Autodesk Inventor part; units mm, degrees
ref_plane "YZ Plane" through (0, 0, 0) normal (1, 0, 0) x (0, 1, 0)
ref_plane "XZ Plane" through (0, 0, 0) normal (0, 1, 0) x (-1, 0, 0)
ref_plane "XY Plane" through (0, 0, 0) normal (0, 0, 1) x (1, 0, 0)
sketch "Sketch4" plane through (0, 0, 0) normal (0, 0, 1) x (1, 0, 0)
  line L0 (-45, -45) -> (45, -45)
  line L1 (45, -45) -> (45, 45)
  line L2 (45, 45) -> (-45, 45)
  line L3 (-45, 45) -> (-45, -45)
  line L4 (-45, -45) -> (45, 45) construction
  line L5 (45, -45) -> (-45, 45) construction
  point P0 (0, 0)
  dimension "d10" = 90
  dimension "d11" = 90
extrude "Extrusion4" add sketch "Sketch4" along normal blind 12.47
sketch "Sketch5" plane through (0, 0, 12.47) normal (0, 0, 1) x (1, 0, 0)
  line L0 (-45, -45) -> (45, -45)
  line L1 (45, -45) -> (45, 45)
  line L2 (45, 45) -> (-45, 45)
  line L3 (-45, 45) -> (-45, -45)
  line L4 (-45, -45) -> (45, 45) construction
  line L5 (45, -45) -> (-45, 45) construction
  line L6 (45, 45) -> (-45, 45)
  line L7 (45, -45) -> (45, 45)
  circle A0 centre (0, 0) radius 40.05
  dimension "d14" = 80.1
extrude "Extrusion5" add sketch "Sketch5" along normal blind 8.1
sketch "Sketch6" plane through (0, 0, 12.47) normal (0, 0, 1) x (1, 0, 0)
  circle A0 centre (0, 0) radius 35
  dimension "d17" = 70
extrude "Extrusion6" cut sketch "Sketch6" against normal through all
sketch "Sketch7" plane through (0, 0, 0) normal (0, 0, -1) x (-1, 0, 0)
  circle A0 centre (0, 0) radius 35
  circle A1 centre (0, 0) radius 35
  circle A2 centre (0, 0) radius 15
  dimension "d20" = 70
  dimension "d21" = 30
extrude "Extrusion7" add sketch "Sketch7" against normal blind 5
sketch "Sketch8" plane through (0, 0, 0) normal (0, 0, -1) x (-1, 0, 0)
  circle A0 centre (-37.5, -12.5) radius 2.05
  circle A1 centre (-37.5, 12.5) radius 2.05
  circle A2 centre (37.5, -12.5) radius 2.05
  circle A3 centre (37.5, 12.5) radius 2.05
  point P0 (0, 0)
hole "Hole1" at (-37.5, -12.5, 0) at (-37.5, 12.5, 0) at (37.5, -12.5, 0) at (37.5, 12.5, 0) direction (0, 0, 1) diameter 4.1 end through all
sketch "Sketch9" plane through (0, 0, 20.57) normal (0, 0, 1) x (1, 0, 0)
  arc A0 (-38.5785, -10.7566) -> (-37.3167, -14.5418) centre (-37.5, -12.5) ccw
  arc A1 (-37.3167, 14.5418) -> (-38.5785, 10.7566) centre (-37.5, 12.5) ccw
  arc A2 (38.5785, 10.7566) -> (37.3167, 14.5418) centre (37.5, 12.5) ccw
  arc A3 (37.3167, -14.5418) -> (38.5785, -10.7566) centre (37.5, -12.5) ccw
  circle A4 centre (-37.5, -12.5) radius 5
  circle A5 centre (-37.5, 12.5) radius 5
  circle A6 centre (37.5, 12.5) radius 5
  circle A7 centre (37.5, -12.5) radius 5
  point P0 (0, 0)
  dimension "d31" = 10
  dimension "d32" = 10
  dimension "d33" = 10
  dimension "d34" = 10
extrude "Extrusion8" cut sketch "Sketch9" against normal blind 15.57
sketch "Sketch10" plane through (0, 0, 20.57) normal (0, 0, 1) x (1, 0, 0)
  circle A0 centre (-37.5, -37.5) radius 2.05
  circle A1 centre (37.5, -37.5) radius 2.05
  circle A2 centre (37.5, 37.5) radius 2.05
  circle A3 centre (-37.5, 37.5) radius 2.05
  circle A4 centre (37.5, -37.5) radius 2.05
  circle A5 centre (-37.5, -37.5) radius 2.05
  line L0 (-45, -45) -> (-45, 45)
  line L1 (-45, 45) -> (45, 45)
  line L2 (45, 45) -> (45, -45)
  line L3 (45, -45) -> (-45, -45)
  circle A6 centre (0, 0) radius 40.05
  point P0 (0, 0)
hole "Hole2" at (-37.5, -37.5, 20.57) at (-37.5, 37.5, 20.57) at (37.5, 37.5, 20.57) at (37.5, -37.5, 20.57) direction (0, 0, -1) diameter 4.1 end through all
sketch "Sketch11" plane through (0, 0, 0) normal (0, 0, -1) x (-1, 0, 0)
  circle A0 centre (37.5, 37.5) radius 2.05
  circle A1 centre (37.5, -37.5) radius 2.05
  circle A2 centre (-37.5, -37.5) radius 2.05
  circle A3 centre (-37.5, 37.5) radius 2.05
  circle A4 centre (37.5, -37.5) radius 5
  circle A5 centre (-37.5, -37.5) radius 5
  circle A6 centre (-37.5, 37.5) radius 5
  circle A7 centre (37.5, 37.5) radius 5
  point P0 (0, 0)
  dimension "d44" = 10
  dimension "d45" = 10
  dimension "d46" = 10
  dimension "d47" = 10
extrude "Extrusion9" cut sketch "Sketch11" against normal blind 5
properties part number "bearing_bracket1" material "ABS Plastic"
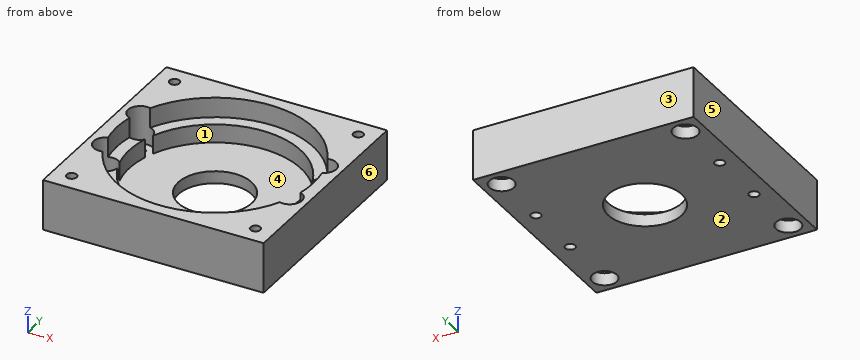
Could you check a few things on this model? Use its own coordinates, in mm. Face numbers are marked on the shaded views. A direction names the side the tool comes from. Give positions to 0.01 mm unless a question says otherwise; leave off trailing zeros. Order: outer loops, then holes, each group sorted by start corner. A loop starts at its lowest first (then second) coordinate and runs counter-clockwise, first axis right, second up. Notation, with made-up numbers: (52, -12) - (71, -12) arc R33 ccw to (71, 26) - close; hole circle Ø10 at (0.5, -11.75). An arc over 180 degrees is marked (long way). Return JSON: item names as keys, results as strings. Group by question number.
Q1. Will these pins go through, and if not, where does the flat tip stop? pin 1 Ø7 at (x, y) = (-36, 4) entering from +Z; pin 2 Ø5 at (x, y) = (-37.5, 38.5) entering from -Z; pin 3 Ø3 at (x, y) = (-28.5, 12) entering from +Z.
Q2. Suppose I cut it at C-C, the plane z = 15.5. Please give me the cut outline in (x, y).
Q3. Which directions (+Z, -Z, +X, -X, +Y, -Y) give clear straight access to the entire face, cutting with the end or side of a thin tool? Please do the marked faces 1 and 2.
Q4. Please list where these lines run through material, in increasing order: line 1 along Y through (x, z) = (37.5, 16.5); line 2 along Y through (x, z) = (37.5, 3.5); line 3 along Y through (x, z) = (37.5, 8.5). Write a range as [from, to].
Q5. Suppose I cut it at A-A, the plane x = 0. Please give me the cut outline in (y, z).
Q6. Suppose I cut it at D-D, the plane y = 37.5. Please give me the cut outline in (x, z), and give its area (3 significant figures).
Q7. Thinking about a two-plate mould opening in X: for the marked faces 3, 4, 5 and 6, which applies, pulls with the +X half, pulls with the -X half, needs draft (parallel to the pull), parting line crosses it, or undercut?
Resolved:
{
 "1": {"pin 1": "stops at z = 12.47", "pin 2": "stops at z = 5", "pin 3": "stops at z = 5"},
 "2": {"outline": "(-45, -45) - (45, -45) - (45, 45) - (-45, 45) - close; hole circle Ø4.1 at (-37.5, -37.5); hole circle Ø4.1 at (-37.5, 37.5); hole (-39.28, -7.83) arc R5 ccw to (-36.12, -17.31) arc R40.05 ccw to (36.12, -17.31) arc R5 ccw to (39.28, -7.83) arc R40.05 ccw to (39.28, 7.83) arc R5 ccw to (36.12, 17.31) arc R40.05 ccw to (-36.12, 17.31) arc R5 ccw to (-39.28, 7.83) arc R40.05 ccw to start; hole circle Ø4.1 at (37.5, -37.5); hole circle Ø4.1 at (37.5, 37.5)"},
 "3": {"face 1": "+Z", "face 2": "-Z, +X, -X, +Y, -Y"},
 "4": {"line 1": "y = [-45, -39.55], [-35.45, -17.5], [17.5, 35.45], [39.55, 45]", "line 2": "y = [-45, -42.5], [-32.5, -14.55], [-10.45, 10.45], [14.55, 32.5], [42.5, 45]", "line 3": "y = [-45, -39.55], [-35.45, -17.5], [-7.5, 7.5], [17.5, 35.45], [39.55, 45]"},
 "5": {"outline": "(-45, 0) - (-15, 0) - (-15, 5) - (-35, 5) - (-35, 12.47) - (-40.05, 12.47) - (-40.05, 20.57) - (-45, 20.57) - close; (15, 0) - (45, 0) - (45, 20.57) - (40.05, 20.57) - (40.05, 12.47) - (35, 12.47) - (35, 5) - (15, 5) - close"},
 "6": {"outline": "(-45, 0) - (-42.5, 0) - (-42.5, 5) - (-39.55, 5) - (-39.55, 20.57) - (-45, 20.57) - close; (-35.45, 5) - (-32.5, 5) - (-32.5, 0) - (32.5, 0) - (32.5, 5) - (35.45, 5) - (35.45, 20.57) - (14.06, 20.57) - (14.06, 12.47) - (-14.06, 12.47) - (-14.06, 20.57) - (-35.45, 20.57) - close; (39.55, 5) - (42.5, 5) - (42.5, 0) - (45, 0) - (45, 20.57) - (39.55, 20.57) - close", "area": "1,400 mm2"},
 "7": {"face 3": "needs draft", "face 4": "undercut", "face 5": "pulls with the -X half", "face 6": "pulls with the +X half"}
}
